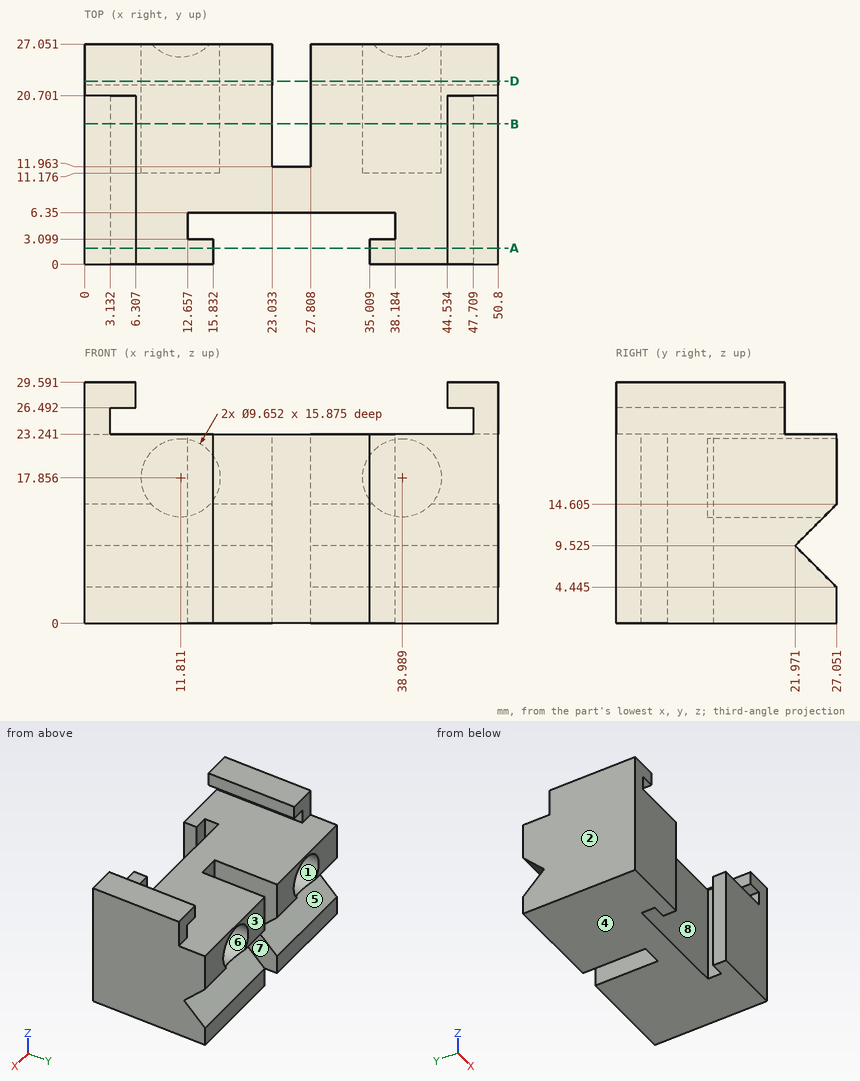
Geometry check sheet. Reference: drawing and pictorial views, mm from the part's lowest x, y, z. A direction names the side the tool comes from. Give positions to 0.01 mm unless a question says otherwise; leave off trailing zeros. Order: outer loops, then holes, each group sorted by start corner. A loop starts at its lowest first (then second) coordinate and runs counter-clockwise, first axis right, second up. Notation, with made-up numbers: M 87.5,-2.5 L 114.5,-2.5 A24 ccw 114.5,17.5 Z; hole C 0,62.25 d5. An arc over 180 degrees is marked long. Answer as CSV lines item,"result". Start each with the question number.
Item 1: Cross-section at A-A on y = 2. Enter the section's corners in (x, z) (1 decimal).
Item 2: Mould release check, pull along X, two halves, no side actions. Record for the marked faces 1, 2 and 3: +X half, -X half, draft (parallel to the pull), parting line (faces both ways), or undercut.
Item 3: Gauge pin test, flat ends, axial feed: P1, Ø3, axis at x = 22, y = 19.5, coming from the +Z side; P2, Ø12, axis at x = 7.5, y = 22, coming from the -Z side; P3, Ø3, axis at x = 4, z = 27, coming from the +Y side; P4, Ø4, axis at x = 25.5, z = 17, coming from the +Y side. Record the tip position at first contact, or that the pin passes through.
Item 4: Thickness scan on line 1 (X direction, y = 6, z = 24.25); line 2 (X direction, y = 6, z = 11) (1 decimal); line 3 (Z direction, x = 46.5, y = 3.5). Record the ranges inside material, lowest first. Write a range as [from, to].
Item 5: Cross-section at D-D on y = 22.5. Enter the section's corners in (x, z).
Item 6: Tool access check on the marked faces 4, 5, 6, 7 and 8. Record the directions out of +Z, -Z, +X, -X, +Y, -Y that give a thin tool (end or side, any length) a straight path to the whole face; none if there is none.
Item 7: Cross-section at B-B on y = 17.25. Enter the section's corners in (x, z) (1 decimal).
Established:
1,outline,"M 0,0 L 15.8,0 L 15.8,23.2 L 3.1,23.2 L 3.1,26.5 L 6.3,26.5 L 6.3,29.6 L 0,29.6 Z; M 35,0 L 50.8,0 L 50.8,29.6 L 44.5,29.6 L 44.5,26.5 L 47.7,26.5 L 47.7,23.2 L 35,23.2 Z"
2,face 1,"undercut"
2,face 2,"-X half"
2,face 3,"draft"
3,P1,"stops at z = 23.24"
3,P2,"stops at z = 0"
3,P3,"stops at y = 20.7"
3,P4,"stops at y = 11.96"
4,line 1,"x = [0, 3.13], [47.71, 50.8]"
4,line 2,"x = [0, 12.7], [38.2, 50.8]"
4,line 3,"z = [0, 23.24], [26.49, 29.59]"
5,outline,"M 0,0 L 23.03,0 L 23.03,9 L 0,9 Z; M 0,10.05 L 23.03,10.05 L 23.03,23.24 L 0,23.24 Z; M 27.81,0 L 50.8,0 L 50.8,9 L 27.81,9 Z; M 27.81,10.05 L 50.8,10.05 L 50.8,23.24 L 27.81,23.24 Z; hole C 11.81,17.86 d9.65; hole C 38.99,17.86 d9.65"
6,face 4,"-Z, +X, -X, +Y, -Y"
6,face 5,"+X, -X, +Y"
6,face 6,"+Y"
6,face 7,"+Z, -Z, +Y"
6,face 8,"+Z, -Z"
7,outline,"M 0,0 L 23,0 L 23,23.2 L 3.1,23.2 L 3.1,26.5 L 6.3,26.5 L 6.3,29.6 L 0,29.6 Z; M 27.8,0 L 50.8,0 L 50.8,29.6 L 44.5,29.6 L 44.5,26.5 L 47.7,26.5 L 47.7,23.2 L 27.8,23.2 Z; hole C 11.8,17.9 d9.7; hole C 39,17.9 d9.7"
